from build123d import *

# Parameters (mm, degrees)
F0_R     = 10
F1_DEPTH = 2
F2_R     = 0.99999
F4_D     = 2


# Not quite as in the source:
# - a fillet or chamfer is up to 0.001 mm smaller than in the source, because OpenCascade refuses the exact size


with BuildPart() as f1:
    # F0 (on Right) → F1 (new body)
    with BuildSketch(Plane.YZ):
        Circle(F0_R)
    extrude(amount=F1_DEPTH)

    # F2 (radius 1 in the source; OpenCascade refuses exactly that, so slightly less here)
    f2_edges = [f1.edges().sort_by_distance(p)[0] for p in [
        (1, 10, 0),
        (0, -10, 0),
        (2, -10, 0),
    ]]
    fillet(f2_edges, radius=F2_R)

    # F4 (through all)
    with Locations(Plane.YZ.offset(2)):
        with Locations((0, 0)):
            Hole(F4_D / 2)


solid = f1.part
Geometry: final body of the model. Coordinates: model frame, mm. Give positions to 0.01 mm unless a question says otherwise; leave off trailing zeros. Loops run counter-clockwise (first coordinate to the right, second up) from the corner with the lowest first, then second, coordinate; pieces in that order, holes last. Notation, with made-up numbers: M 15,65.5 L 20,65.5 A24 ccw 20,101.5 Z; hole C 63,19 d3. An arc over 180 degrees is marked long. Put each result on its own line as item: value. Start each with the question number.
1) Cut plane C-C (x = 0.6). Output: boundary loops of the cut face in (y, z).
2) Contact query for a flat-ended pin moving along its axis: pin 1 (1 mm diameter, centred on x = 1, y = -2, fed in from -Z). Output: stop coordinate, or through.
3) Ray query, line 1 along Z through (x, y) = (1.5, 0); line 2 along Z through (x, y) = (1, 0); line 3 along X through (y, z) = (5.5, 7.75). Return the intervals inside material, ascending.
4) Pull-direction query (Y, two-part tool) for faces 1 (the cylindrical face through (1, 0, -1)), 2 (the flat face through (0, 0, -2)); classes: pulls with the +Y half, pulls with the -Y half, needs draft (parallel to the pull), parting line crosses it, or undercut.
5) Cut plane D-D (x = 1.7). Output: boundary loops of the cut face in (y, z), then the cut area to 3 significant figures.
Verdict:
1. outline: C 0,0 d19.83; hole C 0,0 d2
2. pin 1: z = -9.89
3. line 1: -9.87 to -1, 1 to 9.87
3. line 2: -10 to -1, 1 to 10
3. line 3: 0.14 to 1.86
4. face 1: undercut
4. face 2: needs draft
5. outline: C 0,0 d19.43; hole C 0,0 d2
5. area: 293 mm2
